from build123d import *

# Parameters (mm, degrees)
SKETCH_1_R           = 10
EXTRUDE_1_DEPTH      = 300
M6X1_0_2_D           = 5
M6X1_0_2_DEPTH       = 15
M6X1_0_2_CSINK_D     = 6.05
M6X1_0_2_CSINK_ANGLE = 90
M6X1_0_2_TIP         = 1.502151548
FILLET_1_R           = 1
FILLET_2_R           = 1


with BuildPart() as part:
    # 草图1 → 凸台-拉伸1 (new body)
    with BuildSketch(Plane(origin=(0, 0, 0), x_dir=(1, 0, 0), z_dir=(0, 1, 0))):
        with Locations(Location((0, 0, 0), (0, 0, 270))):
            Circle(SKETCH_1_R)
    extrude(amount=EXTRUDE_1_DEPTH)

    # M6x1.0 螺纹孔2
    with Locations(Plane(origin=(0, 300, 0), x_dir=(1, 0, 0), z_dir=(0, 1, 0))):
        with Locations((0, 0)):
            CounterSinkHole(M6X1_0_2_D / 2, M6X1_0_2_CSINK_D / 2, depth=M6X1_0_2_DEPTH, counter_sink_angle=M6X1_0_2_CSINK_ANGLE)
            with Locations((0, 0, -(M6X1_0_2_DEPTH + M6X1_0_2_TIP / 2))):  # 118° drill point
                Cone(0, M6X1_0_2_D / 2, M6X1_0_2_TIP, mode=Mode.SUBTRACT)

    # 圆角1
    fillet_1_edges = [part.edges().sort_by_distance(p)[0] for p in [
        (0, 300, -10),
    ]]
    fillet(fillet_1_edges, radius=FILLET_1_R)

    # 圆角2
    fillet_2_edges = [part.edges().sort_by_distance(p)[0] for p in [
        (0, 0, -10),
    ]]
    fillet(fillet_2_edges, radius=FILLET_2_R)


solid = part.part
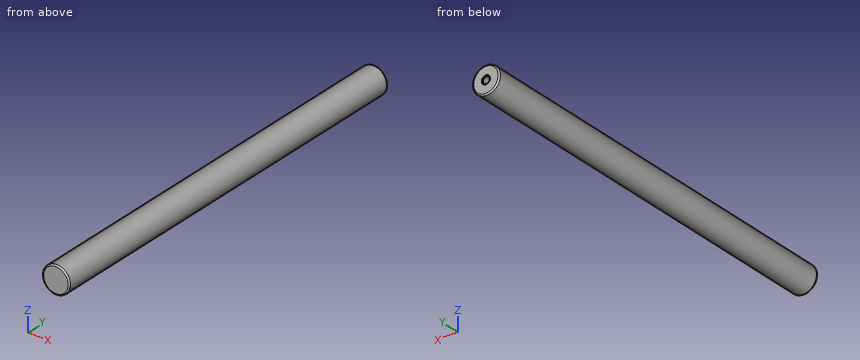
Model file for the job. Use its own axes, mm. Give positions to 0.01 mm unless a question says otherwise; leave off trailing zeros. Order: outer loops, then holes, each group sorted by start corner. A loop starts at its lowest first (then second) coordinate and runs counter-clockwise, first axis right, second up. Notation, with made-up numbers: (17, 4.25) - (51, 4.25) arc R17 ccw to (51, 17.25) - close; hole circle Ø1 at (46, -25). An arc over 180 degrees is marked (long way). Return JSON: item names as keys, results as strings.
1) Cut at A-A, the plane y = 47. Give the cut face in (x, z).
Geometry says:
{"outline": "circle Ø20 at (0, 0)"}
2) Probe line 1 (Y direction, x = -3.25, z = -8.75); line 2 (Z direction, x = 4.25, y = 26.5); line 3 (Y direction, x = 0, z = -3) (3 decimals). List the from-to ranges inside material, lowest first. Write a range as from..to.
Geometry says:
{"line 1": "0.06..299.94", "line 2": "-9.05..9.05", "line 3": "0..299.975"}
3) Flat gauge pins, fed straight in: P1, Ø6, axis at y = 154.5, z = 5, coming from the +X side; P2, Ø1.5, axis at x = -4, y = 205.5, coming from the +Z side; P3, Ø6, axis at y = 209, z = 5, coming from the -X side. Where does each tip first touch, or does it go through?
Geometry says:
{"P1": "x = 9.8", "P2": "z = 9.46", "P3": "x = -9.8"}
